Check sheet for the drawn part. Datum: minimum x, y, z corner. Units: mm. A direction names the side the tool comes from. Round coordinates to 2 decimals unless told otherwise and drop trailing zeros. Write each loop counter-clockwise with the first axis right and the second up, starting at its lowest first coordinate (ties: lowest second). Pieces come first, ordered by that corner, then holes. Notation, with made-up numbers: (2.25, -33) -> (30.25, -33) arc R35 cw to (30.25, 5) -> close; hole circle Ø1 at (54, -17.75). An arc over 180 degrees is marked (long way). One line per item, written item: value.
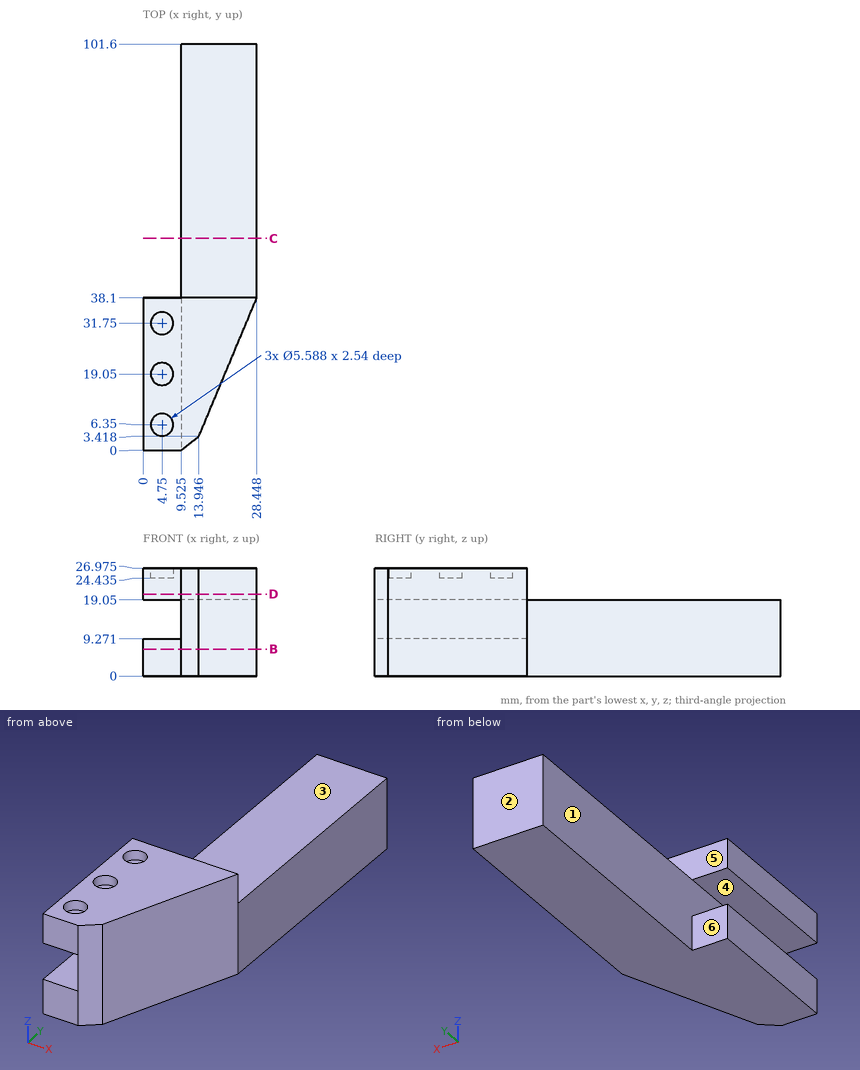
Item 1: Sectioned sample at D-D on z = 20.5. Enter the section's corners in (x, y) (1 decimal).
Answer:
outline: (0, 0) -> (9.5, 0) -> (13.9, 3.4) -> (28.4, 38.1) -> (0, 38.1) -> close
Item 2: Depth check by flat-ended pin: P1, Ø10, axis at x = 5.5, z = 3, coming from the +Y side; P2, Ø8.5, axis at x = 13, z = 23.5, coming from the +Y side; P3, Ø4, axis at y = 42, z = 17.5, coming from the -X side (3 decimals); P4, Ø3, axis at x = 12, z = 15.5, coming from the -Y side. Enter the tip coordinate at first touch or a pass-through.
Answer:
P1: stops at y = 101.6
P2: stops at y = 38.1
P3: stops at x = 9.525
P4: stops at y = 0.75
Item 3: Mould release check, pull along Z, two halves, no side actions. Record for the marked faces 1, 2 and 3: pulls with the +Z half, pulls with the -Z half, needs draft (parallel to the pull), parting line crosses it, or undercut.
Answer:
face 1: undercut
face 2: needs draft
face 3: pulls with the +Z half
Item 4: Sectioned sample at C-C on y = 53. Enter the section's corners in (x, z) (3 decimals).
Answer:
outline: (9.525, 0) -> (28.448, 0) -> (28.448, 19.05) -> (9.525, 19.05) -> close
Item 5: Sectioned sample at B-B on z = 6.75. Enter the section's corners in (x, y) (1 decimal).
Answer:
outline: (0, 0) -> (9.5, 0) -> (13.9, 3.4) -> (28.4, 38.1) -> (28.4, 101.6) -> (9.5, 101.6) -> (9.5, 38.1) -> (0, 38.1) -> close
Item 6: Thickness scan on line 1 (Z direction, x = 17.25, y = 76.5); line 2 (Y direction, x = 2.75, z = 7.25); line 3 (X direction, y = 48, z = 8) (3 decimals). Record the ranges inside material, lowest first.
Answer:
line 1: z = 0 to 19.05
line 2: y = 0 to 38.1
line 3: x = 9.525 to 28.448
Item 7: Tool access check on the marked faces 4, 5 and 6. Record the directions out of +Z, -Z, +X, -X, +Y, -Y that give a thin tool (end or side, any length) a straight path to the whole face; none if there is none.
Answer:
face 4: -X, +Y, -Y
face 5: +Z, +X, -X, +Y
face 6: +Z, -Z, -X, +Y
